CAD build for the part. Positions are in the model's coordinates, mm. A direction names the side the tool comes from. Round coordinates to 2 decimals unless told otherwise and drop trailing zeros. Order: outer loops, then holes, each group sorted by start corner. A loop starts at its lowest first (then second) coordinate and runs counter-clockwise, first axis right, second up. Notation, with made-up numbers: M 40.25,39 L 66.25,39 A12 cw 66.25,59 Z; hole C 28.5,-14 d1. An arc over 180 degrees is marked long. Answer as a JSON object with one key per item and string values. Group by question number.
```python
from build123d import *

# Parameters (mm, degrees)
SKETCH1_R           = 15
BOSS_EXTRUDE1_DEPTH = 25
SKETCH3_W           = 130
SKETCH3_H           = 110
BOSS_EXTRUDE2_DEPTH = 43
SKETCH4_W           = 60
SKETCH4_H           = 110
BOSS_EXTRUDE3_DEPTH = 30
SKETCH5_W           = 42
SKETCH5_H           = 28
CUT_REVOLVE1_ANGLE  = 180
SKETCH6_W           = 56
SKETCH6_H           = 68
CUT_EXTRUDE1_DEPTH  = 15
CUT_EXTRUDE2_DEPTH  = 43


with BuildPart() as part:
    # Sketch1 → Boss-Extrude1 (new body)
    with BuildSketch(Plane(origin=(0, 0, 0), x_dir=(1, 0, 0), z_dir=(0, 1, 0))):
        with BuildLine():
            Line((0, 55), (130, 55))
            Line((130, 55), (130, -55))
            Line((130, -55), (0, -55))
            ThreePointArc((0, -55), (-55, 0), (0, 55))
        make_face()
        Circle(SKETCH1_R, mode=Mode.SUBTRACT)
    extrude(amount=BOSS_EXTRUDE1_DEPTH)

    # Sketch3 → Boss-Extrude2 (add)
    with BuildSketch(Plane(origin=(0, 25, 0), x_dir=(1, 0, 0), z_dir=(0, 1, 0))):
        with Locations((65, 0)):
            Rectangle(SKETCH3_W, SKETCH3_H)
    extrude(amount=BOSS_EXTRUDE2_DEPTH)

    # Sketch4 → Boss-Extrude3 (add)
    with BuildSketch(Plane(origin=(0, 68, 0), x_dir=(1, 0, 0), z_dir=(0, 1, 0))):
        with Locations((30, 0)):
            Rectangle(SKETCH4_W, SKETCH4_H)
    extrude(amount=BOSS_EXTRUDE3_DEPTH)

    # Sketch5 → Cut-Revolve1 (revolve, cut)
    with BuildSketch(Plane.ZY):
        with Locations((-21, 39)):
            Rectangle(SKETCH5_W, SKETCH5_H)
    revolve(axis=Axis((0, 0, 0), (0, -1, 0)), revolution_arc=CUT_REVOLVE1_ANGLE, mode=Mode.SUBTRACT)

    # Sketch6 → Cut-Extrude1 (cut)
    with BuildSketch(Plane(origin=(130, 0, 0), x_dir=(0, 0, -1), z_dir=(1, 0, 0))):
        with Locations((0, 34)):
            Rectangle(SKETCH6_W, SKETCH6_H)
    extrude(amount=-CUT_EXTRUDE1_DEPTH, mode=Mode.SUBTRACT)

    # Sketch7 → Cut-Extrude2 (cut)
    with BuildSketch(Plane(origin=(0, 68, 0), x_dir=(1, 0, 0), z_dir=(0, 1, 0))):
        with BuildLine():
            Line((115, 28), (95, 28))
            ThreePointArc((95, 28), (67, 0), (95, -28))
            Line((95, -28), (115, -28))
            Line((115, -28), (115, 28))
        make_face()
    extrude(amount=-CUT_EXTRUDE2_DEPTH, mode=Mode.SUBTRACT)


solid = part.part
```
Item 1: Flat gauge pins, fed straight in: pin 1 Ø1 at (y, z) = (80.5, -35) entering from +X; pin 2 Ø12.5 at (y, z) = (7.5, 11) entering from +X; pin 3 Ø6 at (y, z) = (44, -21) entering from -X. Where does each tip first touch, or does it go through?
Item 2: Cut at D-D, the plane x = -13. Give the cut face in (y, z).
Item 3: Two-plate mould, pull along Y, no slides. Class faces 1 (the face through (91, 25, 0)), 2 (the face through (113, 41, -28)), 3 (the face through (41.99, 39.2, -0.92)): +Y half, -Y half, draft (parallel to the pull), parting line (faces both ways), or undercut.
Item 4: 3-axis set-ups, long thin cutter, end or side, ignore diameter. For faces 4 (the face through (112, 42, 28)), 5 (the face through (-14.985, 12.325, -0.66)), 6 (the face through (115, 13, 0)): which of +Z, -Z, +X, -X, +Y, -Y reach the whole face in a straight line?
Item 5: Cut at C-C, the plane y = 60. Give the cut face in (x, z), and give its area (3 significant figures).
Item 6: Cut at A-A, the plane z = 0. Give the cut face in (x, y), and give its area (4 significant figures).
Item 7: Drill centre lines: line 1 (X direction, y = 17.25, z = 0); line 2 (Z direction, x = 0, y = 5); line 3 (Z direction, x = 108, y = 57). Where is each one in solid material? Low to high. Write a range as [from, to].
Item 8: Cut at B-B, the plane y = 7. Give the cut face in (x, z).
Response values:
{
 "1": {"pin 1": "x = 60", "pin 2": "x = 115", "pin 3": "x = 34.47"},
 "2": {"outline": "M 0,-53.44 L 25,-53.44 L 25,-7.48 L 0,-7.48 Z; M 0,7.48 L 25,7.48 L 25,53.44 L 0,53.44 Z"},
 "3": {"face 1": "+Y half", "face 2": "draft", "face 3": "undercut"},
 "4": {"face 4": "+X, +Y", "face 5": "-Y", "face 6": "+X, +Y, -Y"},
 "5": {"outline": "M 0,-55 L 130,-55 L 130,-28 L 95,-28 A28 cw 95,28 L 130,28 L 130,55 L 0,55 Z", "area": "11,100 mm^2"},
 "6": {"outline": "M -55,0 L -15,0 L -15,25 L -55,25 Z; M 0,53 L 42,53 L 42,25 L 15,25 L 15,0 L 115,0 L 115,25 L 67,25 L 67,68 L 60,68 L 60,98 L 0,98 Z", "area": "7,005 mm^2"},
 "7": {"line 1": "[-55, -15], [15, 115]", "line 2": "[-55, -15], [15, 55]", "line 3": "[-55, -28], [28, 55]"},
 "8": {"outline": "M 0,-55 L 130,-55 L 130,-28 L 115,-28 L 115,28 L 130,28 L 130,55 L 0,55 A55 ccw Z; hole C 0,0 d30"}
}
